```python
from build123d import *

# Parameters (mm, degrees)
F0_W      = 25.4
F0_H      = 25.4
F1_DEPTH  = 2.794
F2_W      = 19.9765078723
F2_H      = 23.7455442548
F3_DEPTH  = 1.905
F4_R      = 3
F5_DEPTH  = 2.6162
F6_R      = 3.0188611448
F7_DEPTH  = 0.4
F9_DEPTH  = 12.7
F11_D     = 1.27
F11_DEPTH = 12.7
F11_TIP   = 0.3815464931


with BuildPart() as f1:
    # F0 (on Top) → F1 (new body)
    with BuildSketch(Plane.XY):
        Rectangle(F0_W, F0_H)
    extrude(amount=F1_DEPTH)

    # F2 (on Front) → F3 (join, symmetric)
    with BuildSketch(Plane.XZ):
        with Locations((0.2077743411, 11.8727721274)):
            Rectangle(F2_W, F2_H)
    extrude(amount=F3_DEPTH, both=True)

    # F4 (on Front) → F5 (cut, symmetric)
    with BuildSketch(Plane.XZ):
        with Locations((0, 23.7455442548)):
            Circle(F4_R)
    extrude(amount=F5_DEPTH, both=True, mode=Mode.SUBTRACT)

    # F6 (on Front) → F7 (join, symmetric)
    with BuildSketch(Plane.XZ):
        with Locations((0, 23.7644053996)):
            Circle(F6_R)
    extrude(amount=F7_DEPTH, both=True)

    # F8 (on Front) → F9 (cut, symmetric)
    with BuildSketch(Plane.XZ):
        with BuildLine():
            Line((-3.0188022242, 23.7455442548), (-2.7621155605, 23.6954018474))
            ThreePointArc((-2.7621155605, 23.6954018474), (0.0185002573, 20.9847880645), (2.799116075, 23.6954018474))
            Line((2.799116075, 23.6954018474), (3.0188022242, 23.7455442548))
            ThreePointArc((3.0188022242, 23.7455442548), (0, 26.7832665443), (-3.0188022242, 23.7455442548))
        make_face()
    extrude(amount=F9_DEPTH, both=True, mode=Mode.SUBTRACT)

    # F11
    with Locations(Plane.XY.offset(23.7455442548)):
        with Locations((6.3995422242, 0), (-6.3995422242, 0)):
            Hole(F11_D / 2, depth=F11_DEPTH)
            with Locations((0, 0, -(F11_DEPTH + F11_TIP / 2))):  # 118° drill point
                Cone(0, F11_D / 2, F11_TIP, mode=Mode.SUBTRACT)


solid = f1.part
```
For this review, take the finished solid that the model builds, in its own axes (mm). A direction names the side the tool comes from. Round coordinates to 2 decimals unless told otherwise and drop trailing zeros. Write each loop counter-clockwise with the first axis right and the second up, starting at its lowest first coordinate (ties: lowest second). Pieces come first, ordered by that corner, then holes. Notation, with made-up numbers: (49, -19) -> (71, -19) arc R17 ccw to (71, -13) -> close; hole circle Ø3 at (-4, 79.25). An arc over 180 degrees is marked (long way). One line per question, with ' | ' between items. Start each with the question number.
1) Add section C-C (z = 6.5). Write out the cut boundary in (x, y) (3 decimals).
2) Wall thickness on line 1 along X through (y, z) = (0, 14); line 2 along Z through (x, y) = (-3, 11.75); line 3 along Y through (x, z) = (-8.75, 20.25) (3 decimals): over which ranges is each line inside the solid? List them lowest first.
3) For pin 1 Ø5 at (x, y) = (-9, 7) entering from +Z; pin 2 Ø10 at (y, z) = (4, 18.5) entering from +X; pin 3 Ø3.5 at (x, z) = (0.5, 22.5) entering from -Y (3 decimals), all flat-tipped, find the tip position at first contact; note any pin that passes through.
4) Mouldability with a two-part tool opening along Y and no side actions: class faces 6 (the cylindrical face through (6.48, 0.63, 17.31)), 7 (the flat face through (0, 3, 2.794)), 8 (the flat face through (0, 12.7, 1)), 9 (the flat face through (0, -1.905, 13)) as +Y half, -Y half, draft (parallel to the pull), parting line (faces both ways), or undercut.
5) Add section D-D (y = 9.5). Write out the cut boundary in (x, z), and give its area (3 significant figures).
6) Add section A-A (z = 12.25). Write out the cut boundary in (x, y) (3 decimals).
7) Add section B-B (x = -4.5). Write out the cut boundary in (y, z) (3 decimals).
8) Machinability: for faces 1 (the flat face through (0, 1.905, 13)), 2 (the flat face through (-9.78, 0, 13)), 3 (the cylindrical face through (-6.986, -0.243, 17.307)), 4 (the flat face through (10.196, 0, 13)), 5 (the cylindrical face through (-0.066, -1.163, 20.746)), which of the approach directions +Z, -Z, +X, -X, +Y, -Y give a long, thin tool a straight path to every point of the face, cutting with its end or side? Answer none if there is none.
Reported:
1) outline: (-9.78, -1.905) -> (10.196, -1.905) -> (10.196, 1.905) -> (-9.78, 1.905) -> close
2) line 1: x = -9.78 to -7.03, -5.76 to 5.76, 7.03 to 10.2 | line 2: z = 0 to 2.79 | line 3: y = -1.905 to 1.905
3) pin 1: stops at z = 2.79 | pin 2: stops at x = 10.2 | pin 3: stops at y = -1.905
4) face 6: undercut | face 7: draft | face 8: +Y half | face 9: -Y half
5) outline: (-12.7, 0) -> (12.7, 0) -> (12.7, 2.79) -> (-12.7, 2.79) -> close | area: 71.0 mm²
6) outline: (-9.78, -1.905) -> (10.196, -1.905) -> (10.196, 1.905) -> (-9.78, 1.905) -> close; hole circle Ø1.27 at (-6.4, 0); hole circle Ø1.27 at (6.4, 0)
7) outline: (-12.7, 0) -> (12.7, 0) -> (12.7, 2.794) -> (1.905, 2.794) -> (1.905, 23.746) -> (-1.905, 23.746) -> (-1.905, 2.794) -> (-12.7, 2.794) -> close
8) face 1: +Z, +X, -X, +Y | face 2: +Z, -X, +Y, -Y | face 3: +Z | face 4: +Z, +X, +Y, -Y | face 5: +Z, -Y
